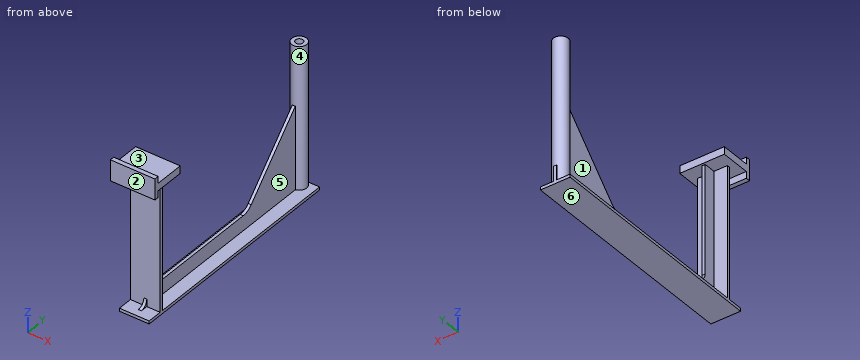
```python
from build123d import *

# Parameters (mm, degrees)
SKETCH1_W                       = 5
SKETCH1_H                       = 20
SKETCH1_W_2                     = 14
SKETCH1_H_2                     = 3
BOSS_EXTRUDE1_DEPTH             = 30
SKETCH4_W                       = 9
SKETCH4_H                       = 2
SKETCH4_W_2                     = 2
SKETCH4_H_2                     = 10
BOSS_EXTRUDE2_DEPTH             = 155
SKETCH4_4_W                     = 2
SKETCH4_4_H                     = 78
BOSS_EXTRUDE3_DEPTH             = 20
SKETCH4_5_W                     = 2
SKETCH4_5_H                     = 10
SKETCH4_5_H_2                   = 78
CUT_EXTRUDE1_DEPTH              = 10
BOSS_EXTRUDE4_REACH             = 184.979
SKETCH2_R                       = 5
SKETCH2_R_2                     = 2.5
BOSS_EXTRUDE4_DIRECTION_2_DEPTH = 5
FILLET1_R                       = 5
BOSS_EXTRUDE6_DEPTH             = 2
FILLET2_R                       = 10
BOSS_EXTRUDE7_DEPTH             = 1
BOSS_EXTRUDE7_DEPTH_BACK        = 1
SKETCH5_W                       = 20
SKETCH5_H                       = 91


with BuildPart() as part:
    # Sketch1 → Boss-Extrude1 (new body)
    with BuildSketch(Plane(origin=(0, 0, 0), x_dir=(0, 0, -1), z_dir=(1, 0, 0))):
        with Locations((0, 11.5)):
            Rectangle(SKETCH1_W, SKETCH1_H)
        Rectangle(SKETCH1_W_2, SKETCH1_H_2)
    extrude(amount=BOSS_EXTRUDE1_DEPTH)



with BuildPart() as body_2:
    # Sketch4 → Boss-Extrude2 (new body)
    with BuildSketch(Plane(origin=(0, 0, 0), x_dir=(1, 0, 0), z_dir=(0, 1, 0))):
        with Locations((20.5, 91.5)):
            Rectangle(SKETCH4_W, SKETCH4_H)
        with Locations((15, 91.5)):
            Rectangle(SKETCH4_W_2, SKETCH4_H)
        with Locations((9.5, 91.5)):
            Rectangle(SKETCH4_W, SKETCH4_H)
        with Locations((15, 85.5)):
            Rectangle(SKETCH4_W_2, SKETCH4_H_2)
    extrude(amount=BOSS_EXTRUDE2_DEPTH)


with BuildPart() as part_1:
    add(part.part)

    add(body_2.part)  # Boss-Extrude3 merges body 2
    # Sketch4<4> → Boss-Extrude3 (add)
    with BuildSketch(Plane(origin=(0, 0, 0), x_dir=(1, 0, 0), z_dir=(0, 1, 0))):
        with Locations((15, 41.5)):
            Rectangle(SKETCH4_4_W, SKETCH4_4_H)
    extrude(amount=BOSS_EXTRUDE3_DEPTH)

    # Sketch4<5> → Cut-Extrude1 (cut)
    with BuildSketch(Plane(origin=(0, 0, 0), x_dir=(1, 0, 0), z_dir=(0, 1, 0))):
        with Locations((15, 85.5)):
            Rectangle(SKETCH4_5_W, SKETCH4_5_H)
        with Locations((15, 41.5)):
            Rectangle(SKETCH4_5_W, SKETCH4_5_H_2)
    extrude(amount=CUT_EXTRUDE1_DEPTH, mode=Mode.SUBTRACT)

    # Boss-Extrude4: up to this face of the body (flat: up to its plane)
    boss_extrude4_end = Plane(part_1.part.faces().sort_by_distance((15, 77.5, -92.5))[0])
    # Sketch2 → Boss-Extrude4 (add, up to the picked face)
    with BuildSketch(Plane.XY, mode=Mode.PRIVATE) as boss_extrude4_sk1:
        with Locations(Location((15, 150, 0), (0, 0, 101.536959033))):
            Circle(SKETCH2_R)
        with Locations(Location((15, 150, 0), (0, 0, 113.578178478))):
            Circle(SKETCH2_R_2, mode=Mode.SUBTRACT)
    boss_extrude4_tool1 = split(extrude(boss_extrude4_sk1.sketch, amount=-BOSS_EXTRUDE4_REACH, mode=Mode.PRIVATE), bisect_by=boss_extrude4_end, keep=Keep.BOTH, mode=Mode.PRIVATE)
    add(boss_extrude4_tool1.solids().sort_by(Axis((15.971716, 145.239585, 0), (0, 0, -1)))[0])

    # Sketch2 → Boss-Extrude4 direction 2 (add)
    with BuildSketch(Plane.XY):
        with Locations(Location((15, 150, 0), (0, 0, 101.536959033))):
            Circle(SKETCH2_R)
        with Locations(Location((15, 150, 0), (0, 0, 113.578178478))):
            Circle(SKETCH2_R_2, mode=Mode.SUBTRACT)
    extrude(amount=BOSS_EXTRUDE4_DIRECTION_2_DEPTH)

    # Fillet1
    fillet1_edges = [part_1.edges().sort_by_distance(p)[0] for p in [
        (15, 20, -80.5),
        (15, 10, -90.5),
    ]]
    fillet(fillet1_edges, radius=FILLET1_R)

    # Sketch6 → Boss-Extrude6 (add)
    with BuildSketch(Plane(origin=(16, 0, 0), x_dir=(0, 0, -1), z_dir=(1, 0, 0))):
        Polygon((80.5, 102), (27.244802727, 152.255197273), (80.5, 152.255197273), align=None)
    extrude(amount=-BOSS_EXTRUDE6_DEPTH)

    # Fillet2
    fillet2_edges = [part_1.edges().sort_by_distance(p)[0] for p in [
        (15, 102, -80.5),
    ]]
    fillet(fillet2_edges, radius=FILLET2_R)

    # Sketch5 → Boss-Extrude7 (add, two sides: drawn at the far end of the back side and taken through both)
    with BuildSketch(Plane(origin=(0, 11, 0), x_dir=(-1, 0, 0), z_dir=(0, -1, 0)).offset(-BOSS_EXTRUDE7_DEPTH_BACK)):
        with Locations((-15, 45)):
            Rectangle(SKETCH5_W, SKETCH5_H)
    extrude(amount=BOSS_EXTRUDE7_DEPTH + BOSS_EXTRUDE7_DEPTH_BACK)


solid = part_1.part
```
Check sheet for the modelled part. Datum: model origin and axes. Units: mm. Face numbers are marked on the shaded views. A direction names the side the tool comes from. Round coordinates to 2 decimals unless told otherwise and drop trailing zeros. Loops run counter-clockwise (first coordinate to the right, second up) from the corner with the lowest first, then second, coordinate; pieces in that order, holes last. Notation, with made-up numbers: (-7, -21) - (12, -21) arc R20 ccw to (12, -6) - close; hole circle Ø7 at (22.5, 13). An arc over 180 degrees is marked (long way). Answer as a JSON object with one key per item and string values. Group by question number.
Q1. Sectioned sample at B-B, the plane y = 85. Enter the section's corners in (x, z), plus the area to 3 significant figures.
Q2. Sectioned sample at C-C, the plane z = -83.5. Enter the section's corners in (x, y).
Q3. Sectioned sample at A-A, the plane z = -46. Enter the section's corners in (x, y), plus the area to 3 significant figures.
Q4. Sectioned sample at D-D, the plane y = 113. Enter the section's corners in (x, z).
Q5. Mould release check, pull along Z, two halves, no side actions. Record for the marked faces 1, 2 and 3: released by +Z, released by -Z, zero draft, split by the parting line, or undercut.
Q6. Scan lines: line 1 along X through (y, z) = (150, -47); line 2 along Y through (x, z) = (15, 2.45); line 3 along X through (y, z) = (150, 1.25). Record each from-to range of solid material in increasing order. Write a range as [from, to].
Q7. Set-up check for the marked faces 4, 5 and 6: record each of +Z, -Z, +X, -X, +Y, -Y from which the full face is reachable in a straight line by a thin tool's end or side.
Q8. Gauge pin test, flat ends, axial feed: P1, Ø1.5, axis at x = 15, y = 107.5, coming from the +Z side; P2, Ø3.5, axis at y = 150.5, z = -51, coming from the -X side; P3, Ø3, axis at x = 21, y = 109, coming from the +Z side. Record the tip position at first contact, or that the pin passes through.
Solution:
{
 "1": {"outline": "(5, -92.5) - (25, -92.5) - (25, -90.5) - (16, -90.5) - (16, -80.5) - (14, -80.5) - (14, -90.5) - (5, -90.5) - close", "area": "60.0 mm²"},
 "2": {"outline": "(5, 10) - (25, 10) - (25, 12) - (16, 12) - (16, 145.1) arc R5 ccw to (16, 154.9) - (16, 155) - (14, 155) - (14, 154.9) arc R5 ccw to (14, 145.1) - (14, 12) - (5, 12) - close; hole (14, 147.71) - (14, 152.29) arc R2.5 ccw to start; hole (16, 147.71) arc R2.5 ccw to (16, 152.29) - close"},
 "3": {"outline": "(5, 10) - (25, 10) - (25, 12) - (16, 12) - (16, 20) - (14, 20) - (14, 12) - (5, 12) - close; (14, 134.56) - (16, 134.56) - (16, 145.1) arc R5 ccw (long way) to (14, 145.1) - close; hole (14, 147.71) - (14, 152.26) - (16, 152.26) - (16, 147.71) arc R2.5 ccw (long way) to start", "area": "145 mm²"},
 "4": {"outline": "(5, -92.5) - (25, -92.5) - (25, -90.5) - (16, -90.5) - (16, -68.84) - (14, -68.84) - (14, -90.5) - (5, -90.5) - close"},
 "5": {"face 1": "undercut", "face 2": "zero draft", "face 3": "released by +Z"},
 "6": {"line 1": "x = [10, 12.5], [14, 16], [17.5, 20]", "line 2": "y = [-1.5, 21.5], [145, 147.5], [152.5, 155]", "line 3": "x = [10, 12.5], [17.5, 20]"},
 "7": {"face 4": "+Z", "face 5": "+X", "face 6": "-Z, +X, -X, +Y, -Y"},
 "8": {"P1": "stops at z = -73.88", "P2": "stops at x = 10", "P3": "stops at z = -90.5"}
}
